Read the model definition and answer for the solid it produces. Units are mm, in the model's axes. Round coordinates to 2 decimals unless told otherwise and drop trailing zeros. Order: outer loops, then holes, each group sorted by start corner. A loop starts at its lowest first (then second) coordinate and runs counter-clockwise, first axis right, second up. Notation, with made-up numbers: M 45.5,72.25 L 87.5,72.25 A32 ccw 87.5,111.25 Z; hole C 11,42.5 d11. An arc over 180 degrees is marked long. Answer as CSV lines item,"result".
```python
from build123d import *

# Parameters (mm, degrees)
F2_DEPTH = 25.4
F3_DEPTH = 25.4
F4_R     = 5.08
F5_R     = 12.827
F5_R_2   = 12.7
F6_DEPTH = 25.4


with BuildPart() as f2:
    # F0 (on Front) → F2 (new body)
    with BuildSketch(Plane.XZ):
        Polygon((-12.7, -16.6841130704), (0, -16.6841130704), (0, 46.8158869296), (-76.2, 46.8158869296), align=None)
        Polygon((0, 46.8158869296), (0, -16.6841130704), (12.7, -16.6841130704), (127, 46.8158869296), align=None)
    extrude(amount=F2_DEPTH)

    # F1 (on face) → F3 (cut)
    with BuildSketch(Plane.XZ):
        with BuildLine():
            ThreePointArc((0, 21.231531626), (-12.7, 8.531531626), (0, -4.168468374))
            Line((0, -4.168468374), (0, 8.531531626))
            Line((0, 8.531531626), (0, 21.231531626))
        make_face()
        with BuildLine():
            Line((0, 8.531531626), (0, -4.168468374))
            ThreePointArc((0, -4.168468374), (8.9802561211, -0.4487244951), (12.7, 8.531531626))
            ThreePointArc((12.7, 8.531531626), (8.9802561211, 17.5117877471), (0, 21.231531626))
            Line((0, 21.231531626), (0, 8.531531626))
        make_face()
    extrude(amount=F3_DEPTH, mode=Mode.SUBTRACT)

    # F4
    f4_edges = [f2.edges().sort_by_distance(p)[0] for p in [
        (-12.7, -12.7, -16.684113),
        (12.7, -12.7, -16.684113),
        (127, -12.7, 46.815887),
        (-76.2, -12.7, 46.815887),
    ]]
    fillet(f4_edges, radius=F4_R)

    # F5 (on face) → F6 (cut)
    with BuildSketch(Plane.XZ.offset(25.4)):
        with Locations((0, 8.531531626)):
            Circle(F5_R)
        with Locations((0, 8.531531626)):
            Circle(F5_R_2, mode=Mode.SUBTRACT)
    extrude(amount=-F6_DEPTH, mode=Mode.SUBTRACT)


solid = f2.part
```
Item 1: A cutting plane is placed at C-C, the plane y = -3.75. Determine the outline of the cut face in (x, z), and give its area (3 significant figures).
Ans:
outline,"M -67.53,38.14 L -14.19,-15.2 A5.08 ccw -10.6,-16.68 L 11.38,-16.68 A5.08 ccw 13.85,-16.04 L 109.86,37.3 A5.08 ccw 107.4,46.82 L -63.94,46.82 A5.08 ccw Z; hole C 0,8.53 d25.65"
area,"6,640 mm2"
Item 2: Determine the mould class of faces 1 (the face through (-41.231, -12.522, 11.847)), 2 (the face through (-2.78, -12.88, -3.99)), 3 (the face through (112.336, -12.878, 42.919)), 4 (the face through (20, -25.4, 23)) for opening direction Z: +Z half, -Z half, draft (parallel to the pull), parting line (faces both ways), or undercut.
Ans:
face 1,"-Z half"
face 2,"undercut"
face 3,"parting line"
face 4,"draft"
Item 3: A cutting plane is placed at D-D, the plane z = -12. Determine the outline of the cut face in (x, y), and give its area (3 significant figures).
Ans:
outline,"M -17.38,-25.4 L 21.13,-25.4 L 21.13,0 L -17.38,0 Z"
area,"978 mm2"
Item 4: Find the intervals of material crossed by probe 1 along Z at (x, y) = (0, -19.25); probe 2 along X at (y, z) = (-22.75, 4.5); probe 3 along X at (y, z) = (-12.25, 14.5), in increasing order. Write a range as [from, to].
Ans:
probe 1,"[-16.68, -4.3], [21.36, 46.82]"
probe 2,"[-33.88, -12.18], [12.18, 50.83]"
probe 3,"[-43.88, -11.35], [11.35, 68.83]"
Item 5: Flat-ended cylindrical pins translate along their axes: pin 1 (12 mm diameter, centred on x = -26, y = -14, fed in from -Z); pin 2 (4 mm diameter, centred on x = 52.5, y = -7, fed in from -Z); pin 3 (2 mm diameter, centred on y = -21, z = 15.5, fed in from +X). Find the tip coordinate at first contact, or state that the pin passes through.
Ans:
pin 1,"z = -9.38"
pin 2,"z = 4.32"
pin 3,"x = 72.43"
Item 6: A cutting plane is placed at A-A, the plane x = 0. Determine the outline of the cut face in (y, z).
Ans:
outline,"M -25.4,-16.68 L 0,-16.68 L 0,-4.3 L -25.4,-4.3 Z; M -25.4,21.36 L 0,21.36 L 0,46.82 L -25.4,46.82 Z"
Item 7: A cutting plane is placed at B-B, the plane z = -1. Determine the outline of the cut face in (x, y), and give its area (3 significant figures).
Ans:
outline,"M -28.38,-25.4 L -8.58,-25.4 L -8.58,0 L -28.38,0 Z; M 8.58,-25.4 L 40.93,-25.4 L 40.93,0 L 8.58,0 Z"
area,"1,320 mm2"
